Design review of the part built by this model. Coordinates are the model's own, in mm. Give positions to 0.01 mm unless a question says otherwise; leave off trailing zeros. Order: outer loops, then holes, each group sorted by start corner. A loop starts at its lowest first (then second) coordinate and runs counter-clockwise, first axis right, second up. Notation, with made-up numbers: (82.25, 7) -> (140.25, 7) arc R16 cw to (140.25, 26) -> close; hole circle Ø6 at (-34.75, -9). An arc over 180 degrees is marked (long way). One line per item, written item: value. Start each with the question number.
1) Consider section A-A (x = -45). State the section outline as (y, z) points, plus the area to 3 significant figures.
2) The part is to be moulded in two halves that separate along X. For faces 1 (the face through (191.93, 1.52, -29.99)), 2 (the face through (51.93, 1.52, -29.99)), 3 (the face through (68, 3, 18)), say which applies: released by +X, released by -X, zero draft, split by the parting line, or undercut.
3) For pin 1 (5 mm diameter, centred on x = -36.5, z = 57.5, fed in from -Y), flat-tipped, find the tip position at first contact; note if it passes through.
4) Consider section C-C (y = 1.35). State how many separate pieces and enclosed holes the cut face has, plus the area to 3 significant figures.
5) Wall thickness on line 1 along Z through (x, y) = (76, 2.75); line 2 along Z through (x, y) = (9, 2.75); line 3 along Z through (x, y) = (153, 0.65): over which ranges is each line inside the solid? List them lowest first. Write a range as from..to.
6) Consider section B-B (x = 59). State the section outline as (y, z) points.
from build123d import *

# Parameters (mm, degrees)
SKETCH_1_W          = 280
SKETCH_1_H          = 150
EXTRUDE_1_DEPTH     = 3
SKETCH_2_W          = 100
SKETCH_2_H          = 16
CUT_EXTRUDE_1_DEPTH = 3
SKETCH_3_W          = 250
SKETCH_3_H          = 5
CUT_EXTRUDE_2_DEPTH = 3
SKETCH_4_R          = 2.5
CUT_EXTRUDE_3_DEPTH = 3
SKETCH_5_W          = 30
SKETCH_5_H          = 30
SKETCH_5_W_2        = 11
CUT_EXTRUDE_4_DEPTH = 3


with BuildPart() as part:
    # 草图1 → 凸台-拉伸1 (new body)
    with BuildSketch(Plane(origin=(0, 0, 0), x_dir=(1, 0, 0), z_dir=(0, 1, 0))):
        with Locations((69.822750754, -35.664148933)):
            Rectangle(SKETCH_1_W, SKETCH_1_H)
    extrude(amount=EXTRUDE_1_DEPTH)

    # 草图2 → 切除-拉伸1 (cut)
    with BuildSketch(Plane(origin=(0, 3, 0), x_dir=(1, 0, 0), z_dir=(0, 1, 0))):
        with Locations((74.822750754, -35.664148933)):
            Rectangle(SKETCH_2_W, SKETCH_2_H)
    extrude(amount=-CUT_EXTRUDE_1_DEPTH, mode=Mode.SUBTRACT)

    # 草图3 → 切除-拉伸2 (cut)
    with BuildSketch(Plane.XZ):
        with Locations((76.910352346, 93.164148933)):
            Rectangle(SKETCH_3_W, SKETCH_3_H)
        with Locations((76.910352346, -21.835851067)):
            Rectangle(SKETCH_3_W, SKETCH_3_H)
    extrude(amount=-CUT_EXTRUDE_2_DEPTH, mode=Mode.SUBTRACT)

    # 草图4 → 切除-拉伸3 (cut)
    with BuildSketch(Plane(origin=(0, 3, 0), x_dir=(1, 0, 0), z_dir=(0, 1, 0))):
        with Locations(Location((-50.177249246, 31.335851067, 0), (0, 0, 270))):
            Circle(SKETCH_4_R)
        with Locations(Location((49.822750754, 31.335851067, 0), (0, 0, 270))):
            Circle(SKETCH_4_R)
        with Locations(Location((189.822750754, 31.335851067, 0), (0, 0, 270))):
            Circle(SKETCH_4_R)
        with Locations(Location((89.822750754, 31.335851067, 0), (0, 0, 270))):
            Circle(SKETCH_4_R)
    extrude(amount=-CUT_EXTRUDE_3_DEPTH, mode=Mode.SUBTRACT)

    # 草图5 → 切除-拉伸4 (cut)
    with BuildSketch(Plane.XZ):
        with Locations((164.822750754, 35.664148933)):
            Rectangle(SKETCH_5_W, SKETCH_5_H)
        with Locations((-34.677249246, 35.664148933)):
            Rectangle(SKETCH_5_W_2, SKETCH_5_H)
    extrude(amount=-CUT_EXTRUDE_4_DEPTH, mode=Mode.SUBTRACT)


solid = part.part
Checked values:
1. outline: (0, -39.34) -> (3, -39.34) -> (3, -24.34) -> (0, -24.34) -> close; (0, -19.34) -> (3, -19.34) -> (3, 90.66) -> (0, 90.66) -> close; (0, 95.66) -> (3, 95.66) -> (3, 110.66) -> (0, 110.66) -> close
1. area: 420 mm^2
2. face 1: undercut
2. face 2: undercut
2. face 3: zero draft
3. pin 1: stops at y = 0
4. separate pieces: 1
4. enclosed holes: 9
4. area: 36,600 mm^2
5. line 1: z = -39.34..-24.34, -19.34..27.66, 43.66..90.66, 95.66..110.66
5. line 2: z = -39.34..-24.34, -19.34..90.66, 95.66..110.66
5. line 3: z = -39.34..-24.34, -19.34..20.66, 50.66..90.66, 95.66..110.66
6. outline: (0, -39.34) -> (3, -39.34) -> (3, -24.34) -> (0, -24.34) -> close; (0, -19.34) -> (3, -19.34) -> (3, 27.66) -> (0, 27.66) -> close; (0, 43.66) -> (3, 43.66) -> (3, 90.66) -> (0, 90.66) -> close; (0, 95.66) -> (3, 95.66) -> (3, 110.66) -> (0, 110.66) -> close
